Input: part model. Units: mm. Frame: model coordinates. A direction names the side the tool comes from. Coordinates: 2 decimals unless noted, no trailing zeros. Loops run counter-clockwise (first coordinate to the right, second up) from the corner with the lowest first, then second, coordinate; pieces in that order, holes last.
```python
from build123d import *

# Parameters (mm, degrees)
F0_R     = 7.5
F0_R_2   = 3
F1_DEPTH = 2
F2_R     = 4.5
F2_R_2   = 3
F3_DEPTH = 0.5
F4_R     = 0.2


with BuildPart() as f1:
    # F0 (on Front) → F1 (new body)
    with BuildSketch(Plane.XZ):
        Circle(F0_R)
        Circle(F0_R_2, mode=Mode.SUBTRACT)
    extrude(amount=F1_DEPTH)

    # F2 (on face) → F3 (join)
    with BuildSketch(Plane.XZ.offset(2)):
        Circle(F2_R)
        Circle(F2_R_2, mode=Mode.SUBTRACT)
    extrude(amount=F3_DEPTH)

    # F4
    f4_edges = [f1.edges().sort_by_distance(p)[0] for p in [
        (-7.5, -2, 0),
        (-7.5, 0, 0),
        (-4.5, -2.5, 0),
    ]]
    fillet(f4_edges, radius=F4_R)


solid = f1.part
```
Item 1: Mould query, pull axis Z, two halves, no side actions, for faces 1 (the face through (0, -2, -5)), 2 (the face through (-3, -1, 0)), 3 (the face through (-7.493, -0.989, 0.33)). Classes: +Z half, -Z half, draft (parallel to the pull), parting line (faces both ways), or undercut.
Result:
face 1: draft
face 2: undercut
face 3: parting line
Item 2: Section query B-B (z = 0). Output: boundary loops of the cut face in (x, y).
Result:
outline: (-7.5, -1.8) arc R0.2 ccw to (-7.3, -2) - (-4.5, -2) - (-4.5, -2.3) arc R0.2 ccw to (-4.3, -2.5) - (-3, -2.5) - (-3, 0) - (-7.3, 0) arc R0.2 ccw to (-7.5, -0.2) - close; (3, -2.5) - (4.3, -2.5) arc R0.2 ccw to (4.5, -2.3) - (4.5, -2) - (7.3, -2) arc R0.2 ccw to (7.5, -1.8) - (7.5, -0.2) arc R0.2 ccw to (7.3, 0) - (3, 0) - close
Item 3: Contact query for a flat-ended pin moving along its axis: P1, Ø1, axis at x = 2.5, y = -1.5, coming from the +Z side. Output: stop coordinate, or through.
Result:
P1: stops at z = 7.23
Item 4: Section query C-C (y = -0.5). Output: boundary loops of the cut face in (x, z), then the cut area to 3 significant figures.
Result:
outline: circle Ø15 at (0, 0); hole circle Ø6 at (0, 0)
area: 148 mm2
Item 5: Section query A-A (x = 0). Output: boundary loops of the cut face in (y, z).
Result:
outline: (-2.5, -4.3) arc R0.2 ccw to (-2.3, -4.5) - (-2, -4.5) - (-2, -7.3) arc R0.2 ccw to (-1.8, -7.5) - (-0.2, -7.5) arc R0.2 ccw to (0, -7.3) - (0, -3) - (-2.5, -3) - close; (-2.5, 3) - (0, 3) - (0, 7.3) arc R0.2 ccw to (-0.2, 7.5) - (-1.8, 7.5) arc R0.2 ccw to (-2, 7.3) - (-2, 4.5) - (-2.3, 4.5) arc R0.2 ccw to (-2.5, 4.3) - close
Item 6: Reachability of faces 4 (the face through (-0.59, -2.15, 4.46)), 5 (the face through (2, 0, -3)) from +Z, -Z, +X, -X, +Y, -Y: full face, straight path, thin tool, end or side. Return the list, or none.
Result:
face 4: -Y
face 5: +Z, -Z, +X, -X, +Y
Item 7: Line query: L1, parallel to Z at x = 0, y = -1.2; L2, parallel to Y at x = 1.5, z = -4.75; L3, parallel to X at y = -0.05, z = -2.5. Output: solid intervals per line, ascending.
Result:
L1: z = -7.5 to -3, 3 to 7.5
L2: y = -2 to 0
L3: x = -7 to -1.66, 1.66 to 7
